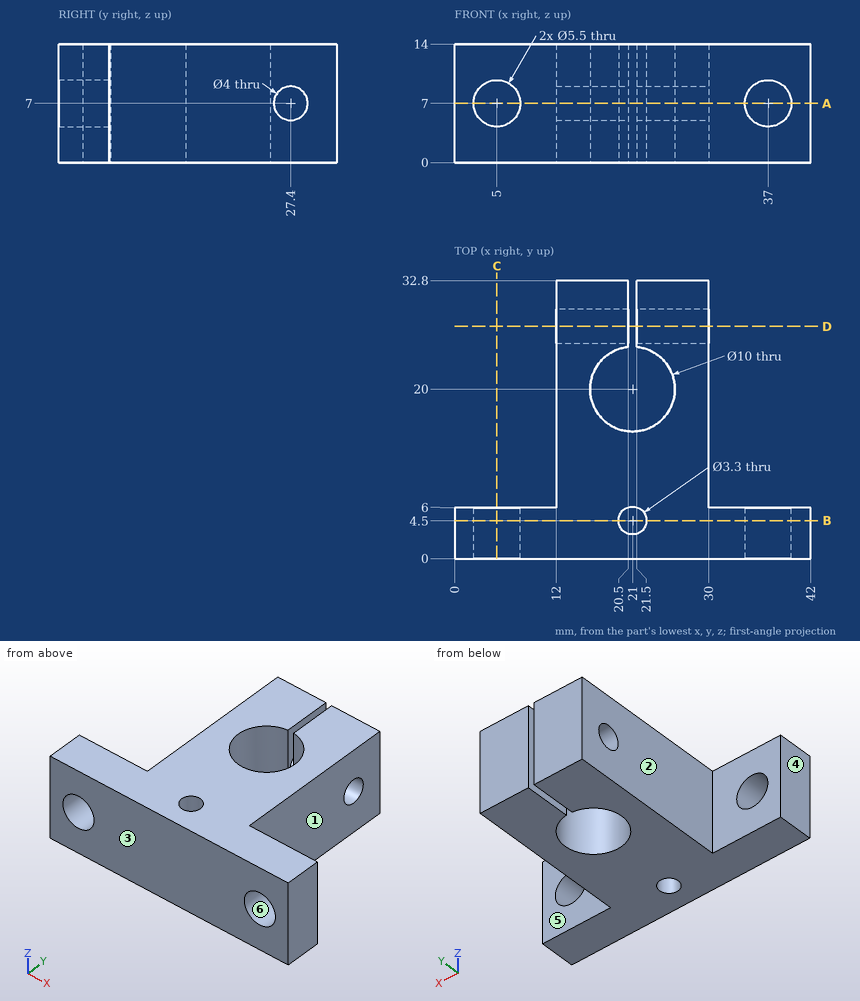
The drawing under review shows one solid part. Ordinate dimensions are in mm from its lowest x, y, z. A direction names the side the tool comes from. Give positions to 0.01 mm unless a question says otherwise; leave off trailing zeros. Write each loop counter-clockwise with the first axis right and the second up, starting at its lowest first coordinate (ties: lowest second). Pieces come first, ordered by that corner, then holes.
1. Draft analysis for pull direction X (two halves, no side actions). For the marked faces 4, 5 and 6, state which applies: +X half, -X half, draft (parallel to the pull), parting line (faces both ways), or undercut.
2. Add section B-B, the plane y = 4.5. Write out the cut boundary in (x, z).
3. Add section D-D, the plane y = 27.4. Write out the cut boundary in (x, z), plus the area to 3 significant figures.
4. Add section A-A, the plane z = 7. Count the separate pieces of the cut face and the enclosed holes in it, plus the area to 4 significant figures.
5. For P1, Ø7, axis at y = 22.5, z = 7.5, coming from the -X side; P2, Ø8, axis at y = 18.5, z = 5.5, coming from the +X side; P3, Ø3, axis at y = 27.4, z = 7, coming from the -X side, all flat-tipped, find the tip position at first contact; note any pin that passes through.
6. Tool access review of the marked faces 1, 2 and 3: name each direction out of +Z, -Z, +X, -X, +Y, -Y from which nothing blocks a thin tool from reaching the whole face with its end or side.
7. Add section C-C, the plane x = 5. Write out the cut boundary in (y, z), plus the area to 3 significant figures.
8. Wall thickness on L1, parallel to Y at x = 21, z = 3.5; L2, parallel to X at y = 31, z = 2; L3, parallel to Z at x = 14, y = 27.4: over which ranges is each line inside the solid? List them lowest first.
Worked answers:
1. face 4: -X half
1. face 5: draft
1. face 6: undercut
2. outline: (0, 0) - (19.35, 0) - (19.35, 14) - (0, 14) - close; (22.65, 0) - (42, 0) - (42, 14) - (22.65, 14) - close; hole circle Ø5.5 at (5, 7); hole circle Ø5.5 at (37, 7)
3. outline: (12, 0) - (20.5, 0) - (20.5, 5) - (12, 5) - close; (12, 9) - (20.5, 9) - (20.5, 14) - (12, 14) - close; (21.5, 0) - (30, 0) - (30, 5) - (21.5, 5) - close; (21.5, 9) - (30, 9) - (30, 14) - (21.5, 14) - close
3. area: 170 mm2
4. separate pieces: 5
4. enclosed holes: 1
4. area: 505.5 mm2
5. P1: stops at x = 12
5. P2: stops at x = 30
5. P3: passes through
6. face 1: +Z, -Z, +X, +Y
6. face 2: +Z, -Z, -X, +Y
6. face 3: +Z, -Z, +X, -X, -Y
7. outline: (0, 0) - (6, 0) - (6, 4.25) - (0, 4.25) - close; (0, 9.75) - (6, 9.75) - (6, 14) - (0, 14) - close
7. area: 51.0 mm2
8. L1: y = 0 to 2.85, 6.15 to 15
8. L2: x = 12 to 20.5, 21.5 to 30
8. L3: z = 0 to 5, 9 to 14
